Here's how the part is built. I have some questions about the finished solid (model axes, mm). A direction names the side the tool comes from. Coordinates: 2 decimals unless noted, no trailing zeros. Order: outer loops, then holes, each group sorted by start corner. A loop starts at its lowest first (then second) coordinate and runs counter-clockwise, first axis right, second up. Notation, with made-up numbers: (-6, 11) - (7, 11) arc R9 cw to (7, 22) - close; hole circle Ø11 at (30.25, -11.75). An arc over 180 degrees is marked (long way). Use CSV: the item, a comma, the result in double quotes. Start each with the question number.
from build123d import *

# Parameters (mm, degrees)
SKETCH1_R           = 1.85
BOSS_EXTRUDE1_DEPTH = 3.1
SKETCH2_R           = 1.5
BOSS_EXTRUDE2_DEPTH = 1
SKETCH3_R           = 1.1
BOSS_EXTRUDE3_DEPTH = 2
SKETCH6_W           = 5
SKETCH6_H           = 5
BOSS_EXTRUDE4_DEPTH = 40
SKETCH7_R           = 1
CUT_EXTRUDE1_DEPTH  = 24


with BuildPart() as part:
    # Sketch1 → Boss-Extrude1 (new body)
    with BuildSketch(Plane(origin=(0, 0, 0), x_dir=(1, 0, 0), z_dir=(0, 1, 0))):
        with Locations(Location((0, 0, 0), (0, 0, 90))):
            Circle(SKETCH1_R)
    extrude(amount=BOSS_EXTRUDE1_DEPTH)

    # Sketch2 → Boss-Extrude2 (add)
    with BuildSketch(Plane(origin=(0, 3.1, 0), x_dir=(1, 0, 0), z_dir=(0, 1, 0))):
        with Locations(Location((0, 0, 0), (0, 0, 270))):
            Circle(SKETCH2_R)
    extrude(amount=BOSS_EXTRUDE2_DEPTH)

    # Sketch3 → Boss-Extrude3 (add)
    with BuildSketch(Plane(origin=(0, 4.1, 0), x_dir=(1, 0, 0), z_dir=(0, 1, 0))):
        with Locations(Location((0, 0, 0), (0, 0, 270))):
            Circle(SKETCH3_R)
    extrude(amount=BOSS_EXTRUDE3_DEPTH)

    # Loft1: read off the stored shape, not the designer's step
    # Loft1: loft between two sections, ruled curve by curve
    loft1_from = [
        Edge.make_bspline([(0, 6.1, 1.85), (3.7, 6.1, 1.85), (3.7, 6.1, -1.85), (0, 6.1, -1.85), (-3.7, 6.1, -1.85), (-3.7, 6.1, 1.85), (0, 6.1, 1.85)], [0, 0, 0, 0, 0.5, 0.5, 0.5, 1, 1, 1, 1], 3, [1, 0.333333333, 0.333333333, 1, 0.333333333, 0.333333333, 1]),
    ]
    loft1_to = [
        Edge.make_bspline([(0.620465421, 8.6, 0.968257539), (2.556980499, 8.6, -0.272673303), (1.316049657, 8.6, -2.209188381), (-0.620465421, 8.6, -0.968257539), (-2.556980499, 8.6, 0.272673303), (-1.316049657, 8.6, 2.209188381), (0.620465421, 8.6, 0.968257539)], [0, 0, 0, 0, 0.5, 0.5, 0.5, 1, 1, 1, 1], 3, [1, 0.333333333, 0.333333333, 1, 0.333333333, 0.333333333, 1]),
    ]
    loft1 = Solid(Shell([*[Face.make_surface_from_curves(loft1_from[k], loft1_to[k]) for k in range(1)], Face(Wire(loft1_from)), Face(Wire(loft1_to))]))
    add(loft1)

    # Sketch6 → Boss-Extrude4 (add)
    with BuildSketch(Plane.XZ):
        Rectangle(SKETCH6_W, SKETCH6_H)
    extrude(amount=BOSS_EXTRUDE4_DEPTH)

    # Sketch7 → Cut-Extrude1 (cut)
    with BuildSketch(Plane.XZ.offset(40)):
        with Locations(Location((0, 0, 0), (0, 0, 270))):
            Circle(SKETCH7_R)
    extrude(amount=-CUT_EXTRUDE1_DEPTH, mode=Mode.SUBTRACT)


solid = part.part
Item 1: For pin 1 Ø1.8 at (x, z) = (0, 0) entering from -Y; pin 2 Ø1.1 at (x, z) = (0, 0.5) entering from -Y, each with a flat end and sliding along its axis, tell me the tip position at first contact or that it passes through.
Item 2: We'd pull the mould along Z, two halves only. Please class faces 5 (the flat face through (0, -20, -2.5)), 6 (the cylindrical face through (-1, -28, 0)), 7 (the flat face through (0, 8.6, 0)): released by +Z, released by -Z, zero draft, split by the parting line, or undercut.
Item 3: Suppose I cut it at A-A on y = -35. Write out the boundary of the cut face in (x, z), then the cut area to 3 significant figures.
Item 4: Please list where these lines run through material, in increasing order: line 1 along X through (y, z) = (-31.25, 0); line 2 along Y through (x, z) = (1.6, -1.1); line 3 along Z through (x, y) = (0.7, -25.5). Write a range as from..to.
Item 5: For faces 1 (the flat face through (1, 0, 2)), 2 (the flat face through (-0.03, -40, 1.15)), 3 (the flat face through (0, -16, 0)), 4 (the cylindrical face through (1.09, 5.09, -0.14)), which set-ups out of +Z, -Z, +X, -X, +Y, -Y let a thin tool reach every point of the face, with its end or its side?
Here are the results:
1,pin 1,"y = -16"
1,pin 2,"y = -40"
2,face 5,"released by -Z"
2,face 6,"undercut"
2,face 7,"zero draft"
3,outline,"(-2.5, -2.5) - (2.5, -2.5) - (2.5, 2.5) - (-2.5, 2.5) - close; hole circle Ø2 at (0, 0)"
3,area,"21.9 mm^2"
4,line 1,"-2.5..-1, 1..2.5"
4,line 2,"-40..0"
4,line 3,"-2.5..-0.71, 0.71..2.5"
5,face 1,"+Y"
5,face 2,"+Z, -Z, +X, -X, -Y"
5,face 3,"-Y"
5,face 4,"none"
